Autodesk Inventor part; units mm, degrees
ref_plane "YZ Plane" through (0, 0, 0) normal (1, 0, 0) x (0, 1, 0)
ref_plane "XZ Plane" through (0, 0, 0) normal (0, 1, 0) x (-1, 0, 0)
ref_plane "XY Plane" through (0, 0, 0) normal (0, 0, 1) x (1, 0, 0)
sketch "Sketch1" plane through (0, 0, 0) normal (0, 0, 1) x (1, 0, 0)
  circle A0 centre (-414.4261, -56.251) radius 4.7625
  point P0 (0, 0)
  dimension "d0" = 9.525
extrude "Extrusion1" add sketch "Sketch1" against normal blind 88.9
sketch "Sketch2" plane through (-414.4261, -56.251, 0) normal (0, 0, 1) x (1, 0, 0)
  circle A0 centre (0, 0) radius 4.7625
  line L0 (-8.2489, 0) -> (-4.1244, 7.1437)
  line L1 (-4.1244, 7.1437) -> (4.1244, 7.1438)
  line L2 (4.1244, 7.1438) -> (8.2489, 0)
  line L3 (8.2489, 0) -> (4.1244, -7.1437)
  line L4 (4.1244, -7.1437) -> (-4.1244, -7.1438)
  line L5 (-4.1244, -7.1438) -> (-8.2489, 0)
  point P0 (414.4261, 56.251)
  dimension "d3" = 14.2875
extrude "Extrusion2" add sketch "Sketch2" along normal blind 3.175 contours A0 | L0 L1 L2 L3 L4 L5
thread "Thread1"
chamfer "Chamfer1" distance 1.016 angle 45 1 edges at (-419.1886, -56.251, -88.9)
properties part number "375 bolt x4" material "Steel"
Here's how the part is built. I have some questions about the finished solid (model axes, mm). A direction names the side the tool comes from. Coordinates: 2 decimals unless noted, no trailing zeros. Order: outer loops, then holes, each group sorted by start corner. A loop starts at its lowest first (then second) coordinate and runs counter-clockwise, first axis right, second up.
1) Imagine slicing it at B-B on x = -420.75. List the corners of the cut face in (y, z) for me (3 decimals), and give its area (3 significant figures).
2) I need wall thicknesses on line 1 (X direction, y = -56.5, z = -28); line 2 (Y direction, x = -414, z = -38.5); line 3 (Z direction, x = -414.5, y = -62.5) (3 decimals). Which ranges of each line are inside material? Lowest first, please.
3) Will these pins go through, and if not, where does the flat tip stop? pin 1 (6 mm diameter, centred on x = -416, z = -72, fed in from -Y); pin 2 (8 mm diameter, centred on y = -51, z = -54.5, fed in from -X); pin 3 (6 mm diameter, centred on y = -52.5, z = -15, fed in from +X).
4) Imagine slicing it at A-A on z = -22. List the corners of the cut face in (x, y) for me (1 decimal).
5) Which directions (+Z, -Z, +X, -X, +Y, -Y) give clear straight access to the entire face, cutting with the end or side of a thin tool? Please do faces 1 (the face through (-408.21, -59.77, 1.57)), 2 (the face through (-415, -51, 0)).
Response values:
1. outline: (-59.585, 0) - (-52.917, 0) - (-52.917, 3.175) - (-59.585, 3.175) - close
1. area: 21.2 mm2
2. line 1: x = -419.18 to -409.67
2. line 2: y = -60.99 to -51.51
2. line 3: z = 0 to 3.175
3. pin 1: stops at y = -61.01
3. pin 2: stops at x = -419.02
3. pin 3: stops at x = -409.72
4. outline: circle Ø9.5 at (-414.4, -56.3)
5. face 1: +Z, -Z, +X, -Y
5. face 2: -Z
